from build123d import *

# Parameters (mm, degrees)
SKETCH_1_W          = 116
SKETCH_1_H          = 53
EXTRUDE_1_DEPTH     = 5
SKETCH_2_W          = 5
SKETCH_2_H          = 53
EXTRUDE_2_DEPTH     = 32
SKETCH_3_R          = 21.5
CUT_EXTRUDE_1_DEPTH = 125.608386556
SKETCH_4_R          = 5
EXTRUDE_3_DEPTH     = 12


with BuildPart() as part:
    # 草图1 → 凸台-拉伸1 (new body)
    with BuildSketch(Plane.XY):
        Rectangle(SKETCH_1_W, SKETCH_1_H)
    extrude(amount=EXTRUDE_1_DEPTH)

    # 草图2 → 凸台-拉伸2 (add)
    with BuildSketch(Plane.XY.offset(5)):
        with Locations((-55.5, 0)):
            Rectangle(SKETCH_2_W, SKETCH_2_H)
    extrude_2 = extrude(amount=EXTRUDE_2_DEPTH)

    # 镜向1: 凸台-拉伸2 across plane
    add(extrude_2.mirror(Plane(origin=(0, 0, 0), x_dir=(0, 0, 1), z_dir=(1, 0, 0))))

    # 草图3 → 切除-拉伸1 (cut, through all)
    with BuildSketch(Plane.ZY.offset(58)):
        with Locations((37, 0)):
            Circle(SKETCH_3_R)
    extrude(amount=-CUT_EXTRUDE_1_DEPTH, mode=Mode.SUBTRACT)

    # 草图4 → 凸台-拉伸3 (add)
    with BuildSketch(Plane(origin=(0, 0, 0), x_dir=(-1, 0, 0), z_dir=(0, 0, -1))):
        with Locations(Location((0, 0, 0), (0, 0, 180))):
            Circle(SKETCH_4_R)
    extrude(amount=EXTRUDE_3_DEPTH)


solid = part.part
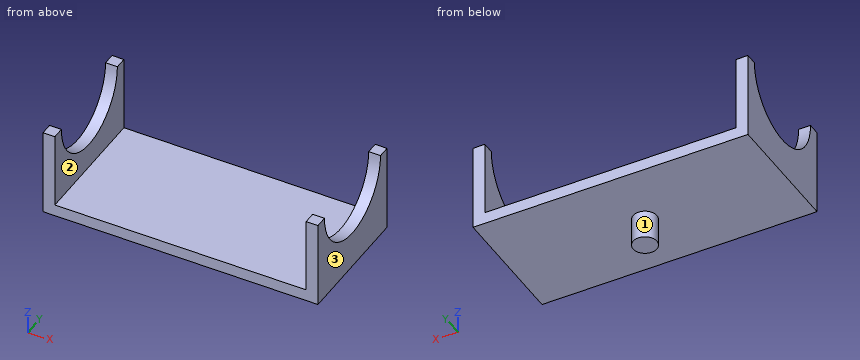
Part model, mm, in its own coordinate system. Face numbers are marked on the shaded views. A direction names the side the tool comes from. Coordinates: 2 decimals unless noted, no trailing zeros. Loops run counter-clockwise (first coordinate to the right, second up) from the corner with the lowest first, then second, coordinate; pieces in that order, holes last. Notation, with made-up numbers: M -22.5,43 L 19.5,43 A31 cw 19.5,70 Z; hole C -27.5,14.25 d5. An arc over 180 degrees is marked long. Use a Markdown table: item, result. Add a question column.
Q1. Cut at B-B (x = 3). Write the cut outline in (y, z).
Q2. Probe L1, parallel to X at y = -10.5, z = 15; L2, parallel to Z at x = -52, y = -22.5. List the from-to ranges inside material, lowest first.
Q3. Which spindle directions (+Z, -Z, +X, -X, +Y, -Y) get a long thin tool onto all of the face, cutting with end or side? Do the marked faces 1, 2 and 3. Say none if no direction does.
Q4. Cut at A-A (y = -17.5). Write the cut outline in (x, z), and give its area (3 significant figures).
Q5. Pin check, flat tip, straight feed: P1, Ø8, axis at x = 0.5, y = -6.5, coming from the +Z side. Stop position of the tip, or through.
Q6. Cut at D-D (x = 34). Write the cut outline in (y, z), and give its area (3 significant figures).
Q7. Cut at C-C (y = 0). Write the cut outline in (x, z), and give its area (3 significant figures).
Worked out:
| question | item | result |
|---|---|---|
| 1 | outline | M -26.5,0 L -4,0 L -4,-12 L 4,-12 L 4,0 L 26.5,0 L 26.5,5 L -26.5,5 Z |
| 2 | L1 | x = -58 to -53, 53 to 58 |
| 2 | L2 | z = 0 to 5 |
| 3 | face 1 | -Z |
| 3 | face 2 | +Z, +Y, -Y |
| 3 | face 3 | +Z, -Z, +X, +Y, -Y |
| 4 | outline | M -58,0 L 58,0 L 58,24.51 L 53,24.51 L 53,5 L -53,5 L -53,24.51 L -58,24.51 Z |
| 4 | area | 775 mm2 |
| 5 | P1 | stops at z = 5 |
| 6 | outline | M -26.5,0 L 26.5,0 L 26.5,5 L -26.5,5 Z |
| 6 | area | 265 mm2 |
| 7 | outline | M -58,0 L -5,0 L -5,-12 L 5,-12 L 5,0 L 58,0 L 58,15.5 L 53,15.5 L 53,5 L -53,5 L -53,15.5 L -58,15.5 Z |
| 7 | area | 805 mm2 |
